Source: CAD feature listing. Evaluate the final solid. Frame: model axes, mm. Face numbers are marked on the shaded views. Round coordinates to 2 decimals unless told otherwise and drop trailing zeros. Write each loop counter-clockwise with the first axis right and the second up, starting at its lowest first coordinate (ties: lowest second). Pieces come first, ordered by that corner, then holes.
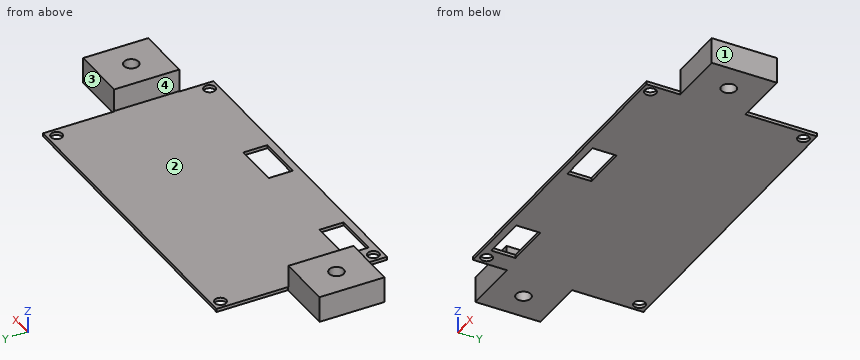
```python
from build123d import *

# Parameters (mm, degrees)
SKIZZE1_R                       = 1.75
SKIZZE1_W                       = 13.916164063
SKIZZE1_H                       = 7.413667428
SKIZZE1_W_2                     = 14.158947343
AUFSATZ_LINEAR_AUSTRAGEN1_DEPTH = 1
SKIZZE2_W                       = 17.347708731
SKIZZE2_H                       = 20
AUFSATZ_LINEAR_AUSTRAGEN2_DEPTH = 7
SKIZZE3_R                       = 2.25
SCHNITT_LINEAR_AUSTRAGEN1_DEPTH = 9


with BuildPart() as part:
    # Skizze1 → Aufsatz-Linear austragen1 (new body)
    with BuildSketch(Plane.XY):
        Polygon((0, 0), (97, 0), (97, 10.4), (114.547708731, 10.4), (114.547708731, 30.4), (97, 30.4), (97, 52.4), (0, 52.4), (0, 30.4), (-17.547708731, 30.4), (-17.547708731, 10.4), (0, 10.4), align=None)
        with Locations((94.3, 49.7)):
            Circle(SKIZZE1_R, mode=Mode.SUBTRACT)
        with Locations((94.3, 2.7)):
            Circle(SKIZZE1_R, mode=Mode.SUBTRACT)
        with Locations((2.7, 2.7)):
            Circle(SKIZZE1_R, mode=Mode.SUBTRACT)
        with Locations((2.7, 49.7)):
            Circle(SKIZZE1_R, mode=Mode.SUBTRACT)
        with Locations((13.256540885, 5.892760701)):
            Rectangle(SKIZZE1_W, SKIZZE1_H, mode=Mode.SUBTRACT)
        with Locations((55.796081341, 5.892760701)):
            Rectangle(SKIZZE1_W_2, SKIZZE1_H, mode=Mode.SUBTRACT)
    extrude(amount=AUFSATZ_LINEAR_AUSTRAGEN1_DEPTH)

    # Skizze2 → Aufsatz-Linear austragen2 (add)
    with BuildSketch(Plane.XY.offset(1)):
        with Locations((-8.873854365, 20.4)):
            Rectangle(SKIZZE2_W, SKIZZE2_H)
        with Locations((105.873854365, 20.4)):
            Rectangle(SKIZZE2_W, SKIZZE2_H)
    extrude(amount=AUFSATZ_LINEAR_AUSTRAGEN2_DEPTH)

    # Skizze3 → Schnitt-Linear austragen1 (cut, through all)
    with BuildSketch(Plane.XY.offset(8)):
        with Locations((-8.873854365, 20.4)):
            Circle(SKIZZE3_R)
        with Locations((105.873854365, 20.4)):
            Circle(SKIZZE3_R)
    extrude(amount=-SCHNITT_LINEAR_AUSTRAGEN1_DEPTH, mode=Mode.SUBTRACT)


solid = part.part
```
Q1. Mould query, pull axis X, two halves, no side actions, for the marked faces 1, 2, 3 and 4. Classes: pulls with the +X half, pulls with the -X half, needs draft (parallel to the pull), parting line crosses it, or undercut.
Q2. Line query: line 1 (Y direction, x = 94.3, z = 0.6); line 2 (Z direction, x = 80, y = 34.5); line 3 (X direction, y = 30, z = 6.75). Output: solid intervals per line, ascending.
Q3. Section query B-B, the plane z = 5. Output: boundary loops of the cut face in (x, y).
Q4. Section query C-C, the plane x = 57. Output: boundary loops of the cut face in (y, z).
Q5. Section query D-D, the plane x = 94.3. Output: boundary loops of the cut face in (y, z).
Q6. Section query A-A, the plane y = 6. Output: boundary loops of the cut face in (x, z).
Q7. Pin query (flat end, axial travel): P1, Ø4.5, axis at x = 2.7, y = 2.7, coming from the +Z side; P2, Ø0.8, axis at y = 6, z = 0.5, coming from the +X side; P3, Ø2, axis at x = 2.7, y = 49.7, coming from the +Z side; P4, Ø1.1, axis at y = 39, z = 0.5, coming from the -X side. Return the tip coordinate at first contact, or that it passes through.
Filled in:
1. face 1: pulls with the +X half
1. face 2: undercut
1. face 3: needs draft
1. face 4: undercut
2. line 1: y = 0 to 0.95, 4.45 to 47.95, 51.45 to 52.4
2. line 2: z = 0 to 1
2. line 3: x = -17.55 to -0.2, 97.2 to 114.55
3. outline: (-17.55, 10.4) - (-0.2, 10.4) - (-0.2, 30.4) - (-17.55, 30.4) - close; (97.2, 10.4) - (114.55, 10.4) - (114.55, 30.4) - (97.2, 30.4) - close; hole circle Ø4.5 at (-8.87, 20.4); hole circle Ø4.5 at (105.87, 20.4)
4. outline: (0, 0) - (2.19, 0) - (2.19, 1) - (0, 1) - close; (9.6, 0) - (52.4, 0) - (52.4, 1) - (9.6, 1) - close
5. outline: (0, 0) - (0.95, 0) - (0.95, 1) - (0, 1) - close; (4.45, 0) - (47.95, 0) - (47.95, 1) - (4.45, 1) - close; (51.45, 0) - (52.4, 0) - (52.4, 1) - (51.45, 1) - close
6. outline: (0, 0) - (6.3, 0) - (6.3, 1) - (0, 1) - close; (20.21, 0) - (48.72, 0) - (48.72, 1) - (20.21, 1) - close; (62.88, 0) - (97, 0) - (97, 1) - (62.88, 1) - close
7. P1: stops at z = 1
7. P2: stops at x = 97
7. P3: passes through
7. P4: stops at x = 0
